Build history of the part. All positions in model axes, mm. A direction names the side the tool comes from. Round coordinates to 2 decimals unless told otherwise and drop trailing zeros. Write each loop counter-clockwise with the first axis right and the second up, starting at its lowest first coordinate (ties: lowest second). Pieces come first, ordered by that corner, then holes.
from build123d import *

# Parameters (mm, degrees)
BOSS_EXTRUDE3_DEPTH = 2
SKETCH4_W           = 114.3
SKETCH4_H           = 5
BOSS_EXTRUDE4_DEPTH = 15


with BuildPart() as part:
    # Sketch3 → Boss-Extrude3 (new body)
    with BuildSketch(Plane.XY):
        with BuildLine():
            Line((-57.15, 120.65), (57.15, 120.65))
            Line((57.15, 120.65), (57.15, 57.15))
            ThreePointArc((57.15, 57.15), (0, 0), (-57.15, 57.15))
            Line((-57.15, 57.15), (-57.15, 120.65))
        make_face()
    extrude(amount=BOSS_EXTRUDE3_DEPTH)

    # Sketch4 → Boss-Extrude4 (add)
    with BuildSketch(Plane.XY.offset(2)):
        with Locations((0, 118.15)):
            Rectangle(SKETCH4_W, SKETCH4_H)
    extrude(amount=BOSS_EXTRUDE4_DEPTH)


solid = part.part
1) Pin check, flat tips, straight feed: pin 1 Ø5 at (x, z) = (-15, 8) entering from -Y; pin 2 Ø4 at (x, y) = (14, 68.5) entering from +Z. Stop position of each tip, or through.
Results:
pin 1: stops at y = 115.65
pin 2: stops at z = 2
2) Slice it at A-A (x = 0). Write the cut outline in (y, z), plus the area to 3 significant figures.
Results:
outline: (0, 0) - (120.65, 0) - (120.65, 17) - (115.65, 17) - (115.65, 2) - (0, 2) - close
area: 316 mm2
3) Slice it at C-C (z = 12.5). Write the cut outline in (x, y).
Results:
outline: (-57.15, 115.65) - (57.15, 115.65) - (57.15, 120.65) - (-57.15, 120.65) - close
4) Slice it at B-B (y = 78.5). Write the cut outline in (x, z), plus the area to 3 significant figures.
Results:
outline: (-57.15, 0) - (57.15, 0) - (57.15, 2) - (-57.15, 2) - close
area: 229 mm2
5) Wall check: L1, parallel to Z at x = -14, y = 106.5; L2, parallel to Y at x = -6, z = 14.75; L3, parallel to X at y = 33, z = 1.5. Give the ranges that are in metal, low to high.
Results:
L1: z = 0 to 2
L2: y = 115.65 to 120.65
L3: x = -51.8 to 51.8
6) Which spindle directions (+Z, -Z, +X, -X, +Y, -Y) get a long thin tool onto all of the face, cutting with end or side? Do faces 1 (the flat face through (1, 59, 2)), 2 (the flat face through (-1, 118, 17)). Say none if no direction does.
Results:
face 1: +Z, +X, -X, -Y
face 2: +Z, +X, -X, +Y, -Y
7) Slice it at D-D (x = 48). Write the cut outline in (y, z).
Results:
outline: (26.13, 0) - (120.65, 0) - (120.65, 17) - (115.65, 17) - (115.65, 2) - (26.13, 2) - close
